```python
from build123d import *

# Parameters (mm, degrees)
SKETCH1_R           = 4
BOSS_EXTRUDE1_DEPTH = 12
SKETCH2_R           = 0.317566637
SKETCH2_R_2         = 0.388464661
BOSS_EXTRUDE2_DEPTH = 5
SKETCH3_R           = 1.5
FILLET1_R           = 1
FILLET2_R           = 0.5
FILLET3_R           = 0.5


with BuildPart() as part:
    # Sketch1 → Boss-Extrude1 (new body)
    with BuildSketch(Plane(origin=(0, 0, 0), x_dir=(1, 0, 0), z_dir=(0, 1, 0))):
        Circle(SKETCH1_R)
    extrude(amount=BOSS_EXTRUDE1_DEPTH)

    # Sketch2 → Boss-Extrude2 (add)
    with BuildSketch(Plane.XZ):
        with Locations((1.75, 0)):
            Circle(SKETCH2_R)
        with Locations((-1.75, 0)):
            Circle(SKETCH2_R_2)
    extrude(amount=BOSS_EXTRUDE2_DEPTH)

    # Sketch3 → Cut-Revolve1 (revolve, cut)
    with BuildSketch(Plane(origin=(0, 0, 0), x_dir=(0, 0, -1), z_dir=(1, 0, 0))):
        with Locations((5.25, 2)):
            Circle(SKETCH3_R)
    revolve(axis=Axis((0, 22.78154861, 0), (0, -1, 0)), mode=Mode.SUBTRACT)

    # Fillet1
    fillet1_edges = [part.edges().sort_by_distance(p)[0] for p in [
        (-2.828427125, 2.829156198, 2.828427125),
        (-2.828427125, 1.170843802, 2.828427125),
    ]]
    fillet(fillet1_edges, radius=FILLET1_R)

    # Fillet2
    fillet2_edges = [part.edges().sort_by_distance(p)[0] for p in [
        (-4, 12, 0),
    ]]
    fillet(fillet2_edges, radius=FILLET2_R)

    # Fillet3
    fillet3_edges = [part.edges().sort_by_distance(p)[0] for p in [
        (-4, 0, 0),
    ]]
    fillet(fillet3_edges, radius=FILLET3_R)


solid = part.part
```
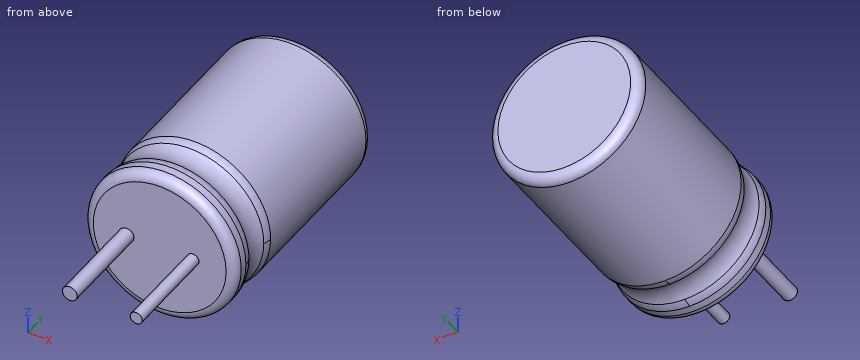
The model under review builds one solid part; all positions refer to its coordinate system, in mm. Give positions to 0.01 mm unless a question says otherwise; leave off trailing zeros. Loops run counter-clockwise (first coordinate to the right, second up) from the corner with the lowest first, then second, coordinate; pieces in that order, holes last. Notation, with made-up numbers: (10, -11.5) - (61, -11.5) arc R25 cw to (61, 2.5) - close; hole circle Ø4 at (67, -17.75). An arc over 180 degrees is marked (long way). Answer as a JSON object with one key per item and string values.
Q1. Add section B-B on y = 8.75. State the section outline as (x, z) points.
Worked out:
{"outline": "circle Ø8 at (0, 0)"}
Q2. To check wall thickness, follow line 1 along Y through (x, z) = (-0.5, 2.5); line 2 along X through (y, z) = (-1.75, -0.25); line 3 along Z through (x, y) = (-3, 6.25). State the ranges of each line that lie inside material, in increasing order.
Worked out:
{"line 1": "y = 0 to 12", "line 2": "x = -2.05 to -1.45, 1.55 to 1.95", "line 3": "z = -2.65 to 2.65"}
Q3. Insertion check: pin 1 (4 mm diameter, centred on x = -1, y = -1.5, fed in from +Z); pin 2 (4 mm diameter, centred on y = 1.5, z = -1.5, fed in from -X); pin 3 (3 mm diameter, centred on x = 1.5, y = 2.5, fed in from -Z). Each pin has a flat end and moves straight along its axis. Give the tip position at first contact, or say it passes through.
Worked out:
{"pin 1": "stops at z = 3.97", "pin 2": "stops at x = -4", "pin 3": "stops at z = -4"}
Q4. Add section A-A on y = -0.5. State the section outline as (x, z) points, plus the area to 3 significant figures.
Worked out:
{"outline": "circle Ø0.78 at (-1.75, 0); circle Ø0.64 at (1.75, 0)", "area": "0.791 mm^2"}
